Autodesk Inventor part; units mm, degrees
ref_plane "YZ Plane" through (0, 0, 0) normal (1, 0, 0) x (0, 1, 0)
ref_plane "XZ Plane" through (0, 0, 0) normal (0, 1, 0) x (-1, 0, 0)
ref_plane "XY Plane" through (0, 0, 0) normal (0, 0, 1) x (1, 0, 0)
sketch "Sketch1" plane through (0, 0, 0) normal (0, 0, 1) x (1, 0, 0)
  line L0 (-264.1156, 220.8859) -> (264.1156, 220.8859)
  line L1 (-264.1156, -220.8859) -> (-264.1156, 220.8859)
  line L2 (264.1156, -220.8859) -> (-264.1156, -220.8859)
  line L3 (264.1156, 220.8859) -> (264.1156, -220.8859)
  line L4 (-207, 203.1016) -> (-207, -132.8984) construction
  line L5 (207, 203.1016) -> (-207, 203.1016) construction
  line L6 (207, -132.8984) -> (207, 203.1016) construction
  line L7 (-207, -132.8984) -> (207, -132.8984) construction
  circle A0 centre (-219.1094, -175.8797) radius 9.5 construction
  circle A1 centre (219.1094, -175.8797) radius 9.5 construction
  circle A2 centre (-219.1094, -175.8797) radius 3.25
  circle A3 centre (219.1094, -175.8797) radius 3.25
  line L8 (-137, 115.1016) -> (169, 115.1016)
  line L9 (169, 115.1016) -> (169, -115.5443)
  line L10 (169, -115.5443) -> (-137, -115.5443)
  line L11 (-137, -115.5443) -> (-137, 115.1016)
  line L12 (159, 103.1016) -> (159, -58.8984)
  line L13 (-127, -24.8984) -> (-127, 105.1016)
  line L14 (-32, 105.1016) -> (-115, 105.1016)
  line L15 (159, 103.1016) -> (159, -58.8984)
  line L16 (159, -58.8984) -> (-6, -58.8984)
  line L17 (-6, -58.8984) -> (-6, 103.1016)
  line L18 (-6, 103.1016) -> (159, 103.1016)
  line L19 (-32, 105.1016) -> (-32, -24.8984)
  line L20 (-32, -24.8984) -> (-127, -24.8984)
  line L21 (-127, -24.8984) -> (-127, 105.1016)
  line L22 (-127, 105.1016) -> (-32, 105.1016)
  line L23 (199, 195.1016) -> (-199, 195.1016)
  line L24 (-199, 195.1016) -> (-199, -130.8984)
  line L25 (-199, -130.8984) -> (199, -130.8984)
  line L26 (199, -130.8984) -> (199, 195.1016)
  circle A4 centre (-254.1156, -114.7989) radius 1
  circle A5 centre (-254.1156, -210.8859) radius 1
  circle A6 centre (-127.0578, -210.8859) radius 1
  circle A7 centre (254.1156, -114.7989) radius 1
  circle A8 centre (254.1156, -210.8859) radius 1
  circle A9 centre (0, -210.8859) radius 1
  circle A10 centre (127.0578, -210.8859) radius 1
  circle A11 centre (-254.1156, 114.7989) radius 1
  circle A12 centre (-254.1156, 0) radius 1
  circle A13 centre (-254.1156, 210.8859) radius 1
  circle A14 centre (-127.0578, 210.8859) radius 1
  circle A15 centre (254.1156, 114.7989) radius 1
  circle A16 centre (127.0578, 210.8859) radius 1
  circle A17 centre (0, 210.8859) radius 1
  circle A18 centre (254.1156, 210.8859) radius 1
  circle A19 centre (254.1156, 0) radius 1
  point P0 (0, 0)
  dimension "d0" = 6.5
  dimension "d1" = 6.5
  dimension "d2" = 10
  dimension "d3" = 10
  dimension "d4" = 10
extrude "Extrusion1" add sketch "Sketch1" along normal blind 6 contours L0 L3 L2 L1 | L8 L9 L10 L11 | L26 L25 L24 L23 | A4 | A5 | A6 | A7 | A8 | A9 | A10 | A11 | A12 | A13 | A14 | A15 | A16 | A17 | A18 | A19
sketch "Sketch2" plane through (0, 0, 6) normal (0, 0, 1) x (1, 0, 0)
  circle A0 centre (-219.1094, -175.8797) radius 3.25 construction
  circle A1 centre (-219.1094, -175.8797) radius 8.5 construction
  point P0 (0, 0)
  point P1 (-219.1094, -167.3797)
  point P2 (-227.6094, -175.8797)
  point P3 (-210.6094, -175.8797)
  point P4 (-219.1094, -184.3797)
  dimension "d7" = 17
hole "Hole1" at (-219.1094, -167.3797, 6) at (-227.6094, -175.8797, 6) at (-210.6094, -175.8797, 6) at (-219.1094, -184.3797, 6) direction (0, 0, -1) diameter 2 end through all
mirror "Mirror1" about plane through (0, 0, 0) normal (1, 0, 0) of "Hole1"
sketch "Sketch3" plane through (0, 0, 6) normal (0, 0, 1) x (1, 0, 0)
  circle A0 centre (-254.1156, 210.8859) radius 1
  circle A1 centre (-127.0578, 210.8859) radius 1
  circle A2 centre (0, 210.8859) radius 1
  circle A3 centre (-254.1156, 114.7989) radius 1
  circle A4 centre (-254.1156, 0) radius 1
  circle A5 centre (127.0578, 210.8859) radius 1
  circle A6 centre (254.1156, 210.8859) radius 1
  circle A7 centre (254.1156, 114.7989) radius 1
  circle A8 centre (254.1156, 0) radius 1
  circle A9 centre (254.1156, -114.7989) radius 1
  circle A10 centre (254.1156, -210.8859) radius 1
  circle A11 centre (127.0578, -210.8859) radius 1
  circle A12 centre (0, -210.8859) radius 1
  circle A13 centre (-127.0578, -210.8859) radius 1
  circle A14 centre (-254.1156, -210.8859) radius 1
  circle A15 centre (-254.1156, -114.7989) radius 1
  point P0 (0, 0)
hole "Hole2" at (-254.1156, 210.8859, 6) at (-127.0578, 210.8859, 6) at (0, 210.8859, 6) at (127.0578, 210.8859, 6) at (254.1156, 210.8859, 6) at (254.1156, 114.7989, 6) at (254.1156, 0, 6) at (254.1156, -114.7989, 6) at (254.1156, -210.8859, 6) at (127.0578, -210.8859, 6) at (0, -210.8859, 6) at (-127.0578, -210.8859, 6) at (-254.1156, -210.8859, 6) at (-254.1156, -114.7989, 6) at (-254.1156, 0, 6) at (-254.1156, 114.7989, 6) direction (0, 0, -1) diameter 3 end through all
properties part number "back"
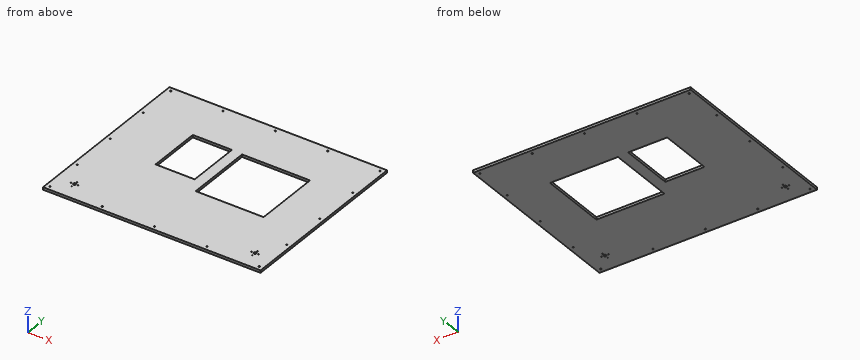
Design review of the part built by this model. Coordinates are the model's own, in mm. Coordinates: 2 decimals unless noted, no trailing zeros. Order: outer loops, then holes, each group sorted by start corner. A loop starts at its lowest first (then second) coordinate and runs counter-clockwise, first axis right, second up. Notation, with made-up numbers: M 86.25,-27 L 128.25,-27 A12 ccw 128.25,-22 Z; hole C 32,44 d10. An arc over 180 degrees is marked long. Answer as a JSON object with one key per item and string values. Group by question number.
1) Add section A-A, the plane x = 50.5. Write out the cut boundary in (y, z), then the cut area to 3 significant figures.
2) Wall thickness on L1, parallel to X at y = -6.5, z = 5.3; L2, parallel to Y at x = 0, z = 2.75; L3, parallel to Y at x = 227.5, z = 0.7: over which ranges is each line inside the solid? List them lowest first.
3) Add section B-B, the plane y = -18.5. Write out the cut boundary in (x, z).
4) Add section C-C, the plane z = 3.8. Count the separate pieces of the cut face and the enclosed holes in it, then the cut area to 3 significant figures.
Computed values:
{
 "1": {"outline": "M -220.89,0 L -58.9,0 L -58.9,6 L -220.89,6 Z; M 103.1,0 L 220.89,0 L 220.89,6 L 103.1,6 Z", "area": "1,680 mm^2"},
 "2": {"L1": "x = -264.12 to -127, -32 to -6, 159 to 264.12", "L2": "y = -220.89 to -212.39, -209.39 to -58.9, 103.1 to 209.39, 212.39 to 220.89", "L3": "y = -220.89 to -176.87, -174.89 to 220.89"},
 "3": {"outline": "M -264.12,0 L -127,0 L -127,6 L -264.12,6 Z; M -32,0 L -6,0 L -6,6 L -32,6 Z; M 159,0 L 264.12,0 L 264.12,6 L 159,6 Z"},
 "4": {"separate pieces": "1", "enclosed holes": "28", "area": "194,000 mm^2"}
}
